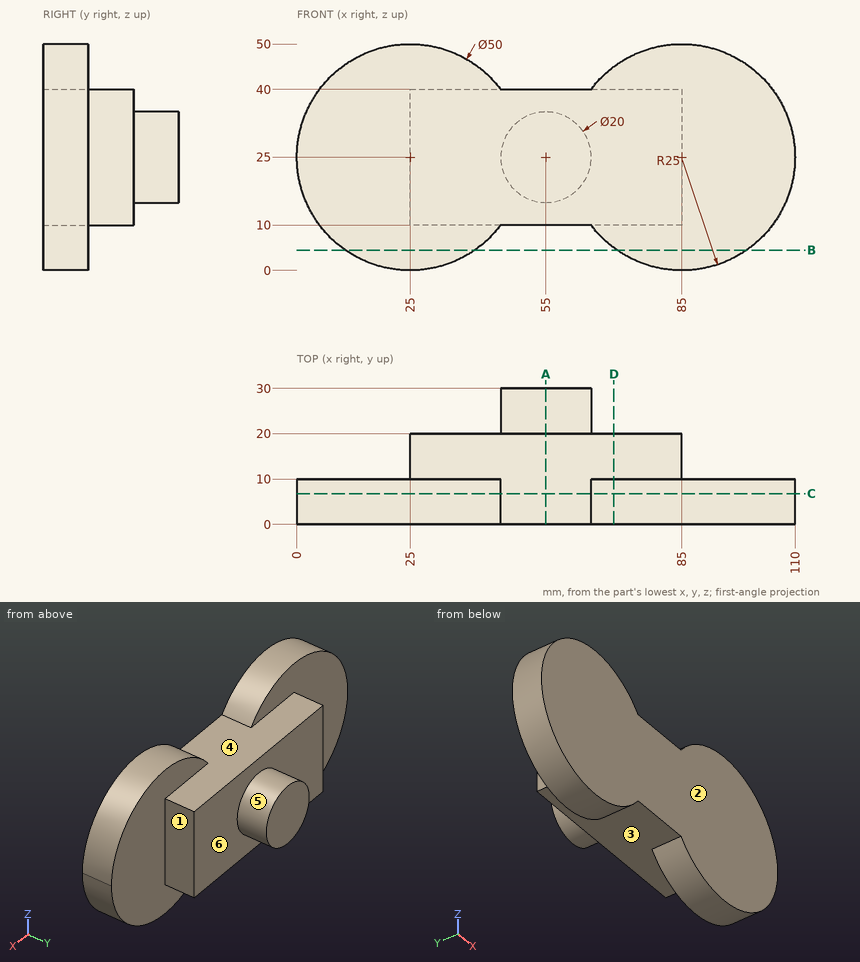
Answer from the drawing. Dimensions are ordinates in mm from the lowest x, y and z of the part. A direction names the side the tool comes from. Give positions to 0.01 mm unless a question says otherwise; leave off trailing zeros. Write each loop counter-clockwise with the first axis right and the second up, starting at its lowest first coordinate (ties: lowest second). Pieces come first, ordered by that corner, then holes. Notation, with made-up numbers: (89.5, 79) -> (148.5, 79) arc R16 ccw to (148.5, 95) -> close; hole circle Ø9 at (69.5, -30.5). An arc over 180 degrees is marked (long way). One line per question, with ' | ' between items. Start each with the question number.
1. Given pin 1 Ø13.5 at (x, z) = (98.5, 29.5) entering from +Y; pin 2 Ø5 at (y, z) = (17.5, 28) entering from -X; pin 3 Ø1.5 at (y, z) = (26, 17) entering from +X, each flat-ended and moving along its own axis, determine where each tip first touches the part or whether it passes through.
2. Section C-C (y = 6.75) is taken. Determine the outline of the cut face in (x, z).
3. Section A-A (x = 55) is taken. Determine the outline of the cut face in (y, z), plus the area to 3 significant figures.
4. For the marked faces 1 and 2, determine the directions among +Z, -Z, +X, -X, +Y, -Y from which every point of the face is accessible in a straight line to the end or side of a thin tool.
5. Section B-B (z = 4.5) is taken. Determine the outline of the cut face in (x, y).
6. Find the intervals of material crossed by probe 1 along Y at (x, z) = (6, 25.5); probe 2 along X at (y, z) = (19.25, 35); probe 3 along Y at (x, z) = (73, 36.5), in increasing order.
7. For a pull along X with two mould halves and no side action, classify the marked faces 3, 4, 5 and 6 as pulls with the +X half, pulls with the -X half, needs draft (parallel to the pull), parting line crosses it, or undercut.
8. Section D-D (x = 70) is taken. Determine the outline of the cut face in (y, z), plus the area to 3 significant figures.
Response values:
1) pin 1: y = 10 | pin 2: x = 25 | pin 3: x = 61.89
2) outline: (45, 10) -> (65, 10) arc R25 ccw (long way) to (65, 40) -> (45, 40) arc R25 ccw (long way) to start
3) outline: (0, 10) -> (20, 10) -> (20, 15) -> (30, 15) -> (30, 35) -> (20, 35) -> (20, 40) -> (0, 40) -> close | area: 800 mm2
4) face 1: +Z, -Z, +X, +Y | face 2: +Z, -Z, +X, -X, -Y
5) outline: (10.69, 0) -> (39.31, 0) -> (39.31, 10) -> (10.69, 10) -> close; (70.69, 0) -> (99.31, 0) -> (99.31, 10) -> (70.69, 10) -> close
6) probe 1: 0 to 10 | probe 2: 25 to 85 | probe 3: 0 to 20
7) face 3: undercut | face 4: undercut | face 5: parting line crosses it | face 6: needs draft
8) outline: (0, 5) -> (10, 5) -> (10, 10) -> (20, 10) -> (20, 40) -> (10, 40) -> (10, 45) -> (0, 45) -> close | area: 700 mm2
